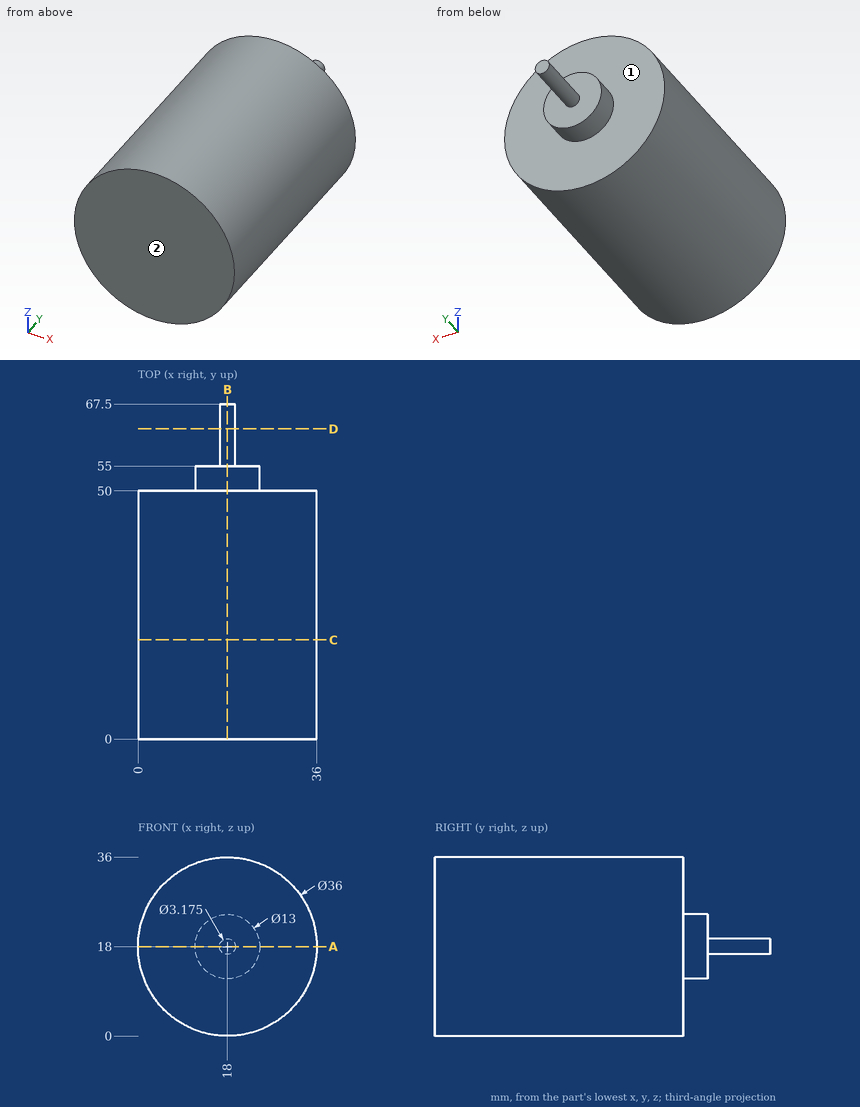
For this review, use the dimensioned drawing (mm, ordinates from the lowest corner) and the shaded views. A direction names the side the tool comes from. Coordinates: 2 decimals unless noted, no trailing zeros. Loops run counter-clockwise (first coordinate to the right, second up) from the corner with the lowest first, then second, coordinate; pieces in that order, holes last.
1. Add section A-A, the plane z = 18. Give the boundary of the cut face in (x, y).
2. Add section D-D, the plane y = 62.5. Give the boundary of the cut face in (x, z) (1 decimal), then the cut area to 3 significant figures.
3. For the marked faces 1 and 2, list the 3-axis set-ups (+Z, -Z, +X, -X, +Y, -Y) from which the entire face can be reached by the end or side of a thin tool; tool diameter is ignored.
4. Add section B-B, the plane x = 18. Give the boundary of the cut face in (y, z).
5. For line 1 (Y direction, x = 32.5, z = 9.5); line 2 (Y direction, x = 13.5, z = 18); line 3 (X direction, y = 15, z = 18.5), list the stretches that pass through material, from the lowest coordinate up.
6. Insertion check: P1, Ø2, axis at x = 25, y = 24.5, coming from the +Z side; P2, Ø10, axis at x = 24, y = 32.5, coming from the +Z side; P3, Ø10, axis at x = 20, y = 27, coming from the -Z side. Each pin has a flat end and moves straight along its axis. Give the tip position at first contact, or say it passes through.
7. Add section C-C, the plane y = 20. Give the boundary of the cut face in (x, z), then the cut area to 3 significant figures.
Result:
1. outline: (0, 0) - (36, 0) - (36, 50) - (24.5, 50) - (24.5, 55) - (19.59, 55) - (19.59, 67.5) - (16.41, 67.5) - (16.41, 55) - (11.5, 55) - (11.5, 50) - (0, 50) - close
2. outline: circle Ø3.2 at (18, 18)
2. area: 7.92 mm2
3. face 1: +Y
3. face 2: +Z, -Z, +X, -X, -Y
4. outline: (0, 0) - (50, 0) - (50, 11.5) - (55, 11.5) - (55, 16.41) - (67.5, 16.41) - (67.5, 19.59) - (55, 19.59) - (55, 24.5) - (50, 24.5) - (50, 36) - (0, 36) - close
5. line 1: y = 0 to 50
5. line 2: y = 0 to 55
5. line 3: x = 0.01 to 35.99
6. P1: stops at z = 34.97
6. P2: stops at z = 35.97
6. P3: stops at z = 0
7. outline: circle Ø36 at (18, 18)
7. area: 1,020 mm2
